```python
from build123d import *

# Parameters (mm, degrees)
F0_W          = 9
F0_H          = 15.2
F1_DEPTH      = 11
F3_DEPTH      = 11.7
F4_R          = 1
F5_DEPTH      = 13
F6_R          = 1.1
F6_W          = 3
F6_H          = 1
F6_W_2        = 1
F6_H_2        = 3
F7_DEPTH      = 3.5
F7_DEPTH_BACK = 1


with BuildPart() as f1:
    # F0 (on Top) → F1 (new body)
    with BuildSketch(Plane.XY):
        Rectangle(F0_W, F0_H)
    extrude(amount=F1_DEPTH)

    # F2 (on face) → F3 (cut)
    with BuildSketch(Plane(origin=(0, 7.6, 0), x_dir=(-1, 0, 0), z_dir=(0, 1, 0))):
        with BuildLine():
            ThreePointArc((-4.5, 6.5), (-3.181981, 9.681981), (0, 11))
            Line((0, 11), (-4.5, 11))
            Line((-4.5, 11), (-4.5, 6.5))
        make_face()
        with BuildLine():
            ThreePointArc((0, 11), (3.181981, 9.681981), (4.5, 6.5))
            Line((4.5, 6.5), (4.5, 11))
            Line((4.5, 11), (0, 11))
        make_face()
    extrude(amount=-F3_DEPTH, mode=Mode.SUBTRACT)

    # F4 (on face) → F5 (cut)
    with BuildSketch(Plane.XZ.offset(7.6)):
        with BuildLine():
            ThreePointArc((2.423324, 5), (2.741256, 5.720248), (2.85, 6.5))
            ThreePointArc((2.85, 6.5), (2.741256, 7.279752), (2.423324, 8))
            ThreePointArc((2.423324, 8), (0, 9.35), (-2.423324, 8))
            ThreePointArc((-2.423324, 8), (-2.85, 6.5), (-2.423324, 5))
            ThreePointArc((-2.423324, 5), (0, 3.65), (2.423324, 5))
        make_face()
        with Locations((0, 6.5)):
            Circle(F4_R, mode=Mode.SUBTRACT)
        with BuildLine():
            ThreePointArc((-2.423324, 5), (-2.85, 6.5), (-2.423324, 8))
            Line((-2.423324, 8), (-3.423324, 8))
            ThreePointArc((-3.423324, 8), (-3.761047, 6.5), (-3.423324, 5))
            Line((-3.423324, 5), (-2.423324, 5))
        make_face()
        with BuildLine():
            ThreePointArc((2.423324, 8), (2.741256, 7.279752), (2.85, 6.5))
            ThreePointArc((2.85, 6.5), (2.741256, 5.720248), (2.423324, 5))
            Line((2.423324, 5), (3.423324, 5))
            ThreePointArc((3.423324, 5), (3.761047, 6.5), (3.423324, 8))
            Line((3.423324, 8), (2.423324, 8))
        make_face()
    extrude(amount=-F5_DEPTH, mode=Mode.SUBTRACT)

    # F6 (on face) → F7 (join, two sides)
    with BuildSketch(Plane(origin=(0, 0, 0), x_dir=(1, 0, 0), z_dir=(0, 0, -1))) as f7_sk:
        with Locations((0, 3.6)):
            Circle(F6_R)
        with Locations((0, -0.9)):
            Rectangle(F6_W, F6_H)
        with Locations((0, -6.9)):
            Rectangle(F6_W, F6_H)
        with Locations((4.7, -3.9)):
            Rectangle(F6_W_2, F6_H_2)
    extrude(amount=F7_DEPTH)
    extrude(f7_sk.sketch, amount=-F7_DEPTH_BACK)


solid = f1.part
```
CAD build for the part. Positions are in the model's coordinates, mm. A direction names the side the tool comes from. Give positions to 0.01 mm unless a question says otherwise; leave off trailing zeros. Order: outer loops, then holes, each group sorted by start corner. A loop starts at its lowest first (then second) coordinate and runs counter-clockwise, first axis right, second up.
(1) Saw through at B-B, the plane z = -0.5. Give the cut face in (x, y).
(2) Saw through at D-D, the plane x = 0.75. Give the cut face in (y, z), then the cut area to 3 significant figures.
(3) Saw through at C-C, the plane y = -0.5. Give the cut face in (x, z), then the cut area to 3 significant figures.
(4) Saw through at A-A, the plane y = -6.25. Give the cut face in (x, z), then the cut area to 3 significant figures.
(5) Drill centre lines: L1, parallel to X at y = 5.75, z = 2.25; L2, parallel to Z at x = 2, y = 2.75; L3, parallel to Y at x = -2.5, z = 6. Where is each one in solid material? Low to high.
(6) Flat gauge pins, fed straight in: pin 1 (3 mm diameter, centred on y = -5.5, z = 9, fed in from +X); pin 2 (0.5 mm diameter, centred on y = 1, z = -2.5, fed in from +X); pin 3 (0.5 mm diameter, centred on y = 1, z = -2, fed in from -X). Where does each tip first touch, or does it go through?
(7) Mould opens along Z. For faces 4 (the flat face through (5, 4, -3.5)), 5 (the flat face through (3, -1, 5)), 6 (the cylindrical face through (-3.76, -1.19, 6.52)), 7 (the flat face through (5, 2.4, -1)) say: released by +Z, released by -Z, zero draft, split by the parting line, or undercut.
(8) Tool access for faces 1 (the flat face through (1.5, 7, -2)), 2 (the flat face through (3, -1, 8)), 3 (the flat face through (-3.4, -4.1, 10.1)): list every direction of +Z, -Z, +X, -X, +Y, -Y with a clear straight run to the whole face (end or side of a thin tool).
Results found:
1. outline: (-1.5, 0.4) - (1.5, 0.4) - (1.5, 1.4) - (-1.5, 1.4) - close; (-1.5, 6.4) - (1.5, 6.4) - (1.5, 7.4) - (-1.5, 7.4) - close; circle Ø2.2 at (0, -3.6); (4.2, 2.4) - (5.2, 2.4) - (5.2, 5.4) - (4.2, 5.4) - close
2. outline: (-7.6, 0) - (-4.4, 0) - (-4.4, -3.5) - (-2.8, -3.5) - (-2.8, 0) - (0.4, 0) - (0.4, -3.5) - (1.4, -3.5) - (1.4, 0) - (6.4, 0) - (6.4, -3.5) - (7.4, -3.5) - (7.4, 0) - (7.6, 0) - (7.6, 10.94) - (-4.1, 10.94) - (-4.1, 11) - (-7.6, 11) - (-7.6, 9.25) - (5.4, 9.25) - (5.4, 7.16) - (-7.6, 7.16) - (-7.6, 5.84) - (5.4, 5.84) - (5.4, 3.75) - (-7.6, 3.75) - close
2. area: 125 mm2
3. outline: (-4.5, 0) - (4.5, 0) - (4.5, 6.5) arc R4.5 ccw to (0, 11) arc R4.5 ccw to (-4.5, 6.5) - close; circle Ø2 at (0, 6.5); hole (-3.42, 5) - (-2.42, 5) arc R2.85 ccw to (2.42, 5) - (3.42, 5) arc R3.5 ccw to (3.42, 8) - (2.42, 8) arc R2.85 ccw to (-2.42, 8) - (-3.42, 8) arc R3.5 ccw to start
3. area: 62.3 mm2
4. outline: (-4.5, 0) - (4.5, 0) - (4.5, 11) - (-4.5, 11) - close; circle Ø2 at (0, 6.5); hole (-3.42, 5) - (-2.42, 5) arc R2.85 ccw to (2.42, 5) - (3.42, 5) arc R3.5 ccw to (3.42, 8) - (2.42, 8) arc R2.85 ccw to (-2.42, 8) - (-3.42, 8) arc R3.5 ccw to start
4. area: 71.0 mm2
5. L1: x = -4.5 to 4.5
5. L2: z = 0 to 4.47, 8.53 to 10.53
5. L3: y = 5.4 to 7.6
6. pin 1: stops at x = 4.5
6. pin 2: stops at x = 1.5
6. pin 3: stops at x = -1.5
7. face 4: released by -Z
7. face 5: undercut
7. face 6: undercut
7. face 7: zero draft
8. face 1: -Z, +X, +Y, -Y
8. face 2: -Y
8. face 3: +Z, -X, +Y
